Input: dimensioned drawing with shaded views. Units: mm. Origin: part minimum x, y, z. A direction names the side the tool comes from. Round coordinates to 2 decimals unless told otherwise and drop trailing zeros. Write each loop counter-clockwise with the first axis right and the second up, starting at its lowest first coordinate (ties: lowest second). Pieces come first, ordered by that corner, then holes. Notation, with made-up numbers: (78, 81) -> (108, 81) arc R29 cw to (108, 114) -> close; hole circle Ø2 at (70.5, 80). An arc over 180 degrees is marked (long way). One line per item, written item: value. Start each with the question number.
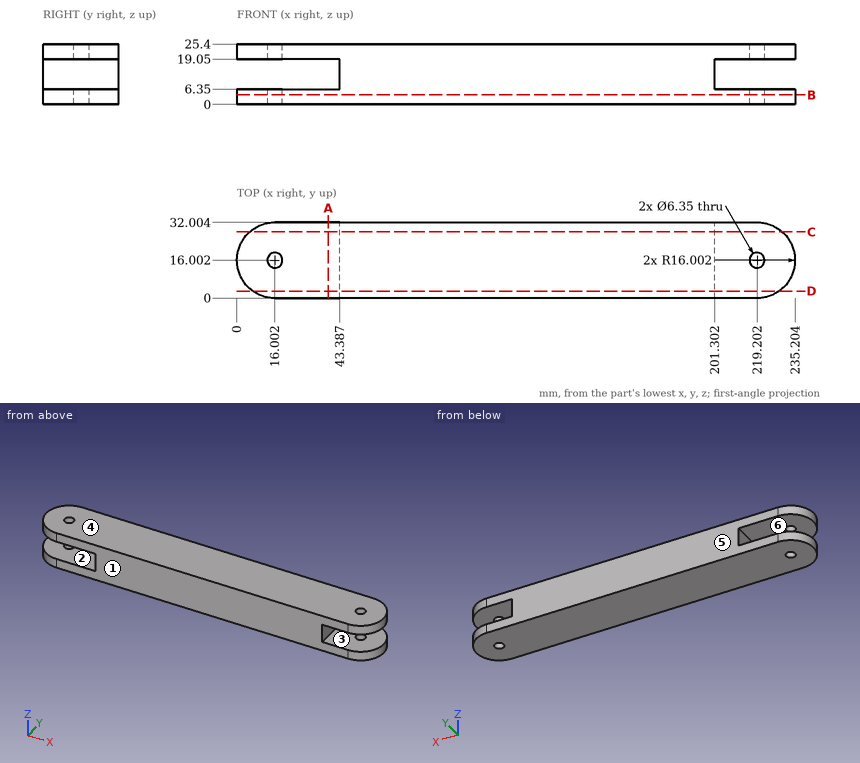
(1) Section query C-C (y = 28). Output: boundary loops of the cut face in (x, z), and give its area (4 significant figures).
(2) Line query: probe 1 along Z at (x, y) = (210, 24); probe 2 along X at (y, z) = (15, 11); probe 3 along X at (y, z) = (28.5, 23.75) (1 decimal). Output: solid intervals per line, ascending.
(3) Section query B-B (z = 4). Output: boundary loops of the cut face in (x, y) (3 decimals), and give its area (3 significant figures).
(4) Section query D-D (y = 3). Output: boundary loops of the cut face in (x, z).
(5) Pin query (flat end, axial travel): pin 1 (12 mm diameter, centred on y = 4, z = 9, fed in from -X); pin 2 (5.5 mm diameter, centred on x = 16.002, y = 16.002, fed in from -Z); pin 3 (5 mm diameter, centred on y = 13.5, z = 14, fed in from +X); pin 4 (4 mm diameter, centred on y = 17.5, z = 14.5, fed in from -X). Return the tip coordinate at first contact, or that it passes through.
(6) Pull-direction query (Z, two-part tool) for the marked faces 4, 5 and 6; classes: pulls with the +Z half, pulls with the -Z half, needs draft (parallel to the pull), parting line crosses it, or undercut.
(7) Set-up query: the marked faces 1, 2 and 3. Return all of +Z, -Z, +X, -X, +Y, -Y with unobstructed straight access to the full face (end or side cutting, diameter ignored); none if empty.
(8) Section query A-A (x = 38.5). Output: boundary loops of the cut face in (y, z).
Results list:
1. outline: (5.41, 0) -> (229.79, 0) -> (229.79, 6.35) -> (201.3, 6.35) -> (201.3, 19.05) -> (229.79, 19.05) -> (229.79, 25.4) -> (5.41, 25.4) -> (5.41, 19.05) -> (43.39, 19.05) -> (43.39, 6.35) -> (5.41, 6.35) -> close
1. area: 4,855 mm^2
2. probe 1: z = 0 to 6.35, 19.05 to 25.4
2. probe 2: x = 43.39 to 201.3
2. probe 3: x = 6 to 229.2
3. outline: (16.002, 0) -> (219.202, 0) arc R16.002 ccw to (219.202, 32.004) -> (16.002, 32.004) arc R16.002 ccw to start; hole circle Ø6.35 at (16.002, 16.002); hole circle Ø6.35 at (219.202, 16.002)
3. area: 7,240 mm^2
4. outline: (6.67, 0) -> (228.53, 0) -> (228.53, 6.35) -> (201.3, 6.35) -> (201.3, 19.05) -> (228.53, 19.05) -> (228.53, 25.4) -> (6.67, 25.4) -> (6.67, 19.05) -> (43.39, 19.05) -> (43.39, 6.35) -> (6.67, 6.35) -> close
5. pin 1: stops at x = 1.43
5. pin 2: passes through
5. pin 3: stops at x = 201.3
5. pin 4: stops at x = 43.39
6. face 4: pulls with the +Z half
6. face 5: needs draft
6. face 6: undercut
7. face 1: +Z, -Z, +X, -X, -Y
7. face 2: -X, +Y, -Y
7. face 3: +X, +Y, -Y
8. outline: (0, 0) -> (32, 0) -> (32, 6.35) -> (0, 6.35) -> close; (0, 19.05) -> (32, 19.05) -> (32, 25.4) -> (0, 25.4) -> close
